from build123d import *

# Parameters (mm, degrees)
F1_DEPTH = 27.7749
F2_R     = 6.604
F4_D     = 6.604


with BuildPart() as f1:
    # F0 (on Right) → F1 (new body, symmetric)
    with BuildSketch(Plane.YZ):
        Polygon((77.47, 13.716), (0, 8.001), (0, 0), (77.47, 0), align=None)
    extrude(amount=F1_DEPTH, both=True)

    # F2
    f2_edges = [f1.edges().sort_by_distance(p)[0] for p in [
        (27.7749, 0, 4.0005),
        (27.7749, 77.47, 6.858),
        (-27.7749, 77.47, 6.858),
        (-27.7749, 0, 4.0005),
    ]]
    fillet(f2_edges, radius=F2_R)

    # F4 (through all)
    with Locations(Plane(origin=(0, 0, 0), x_dir=(1, 0, 0), z_dir=(0, 0, -1))):
        with Locations((22.0599, -5.715), (-22.0599, -5.715), (22.0599, -71.755), (-22.0599, -70.866)):
            Hole(F4_D / 2)


solid = f1.part
Geometry check sheet. Reference: the model listing, model coordinates, mm. Give positions to 0.01 mm unless a question says otherwise; leave off trailing zeros. Order: outer loops, then holes, each group sorted by start corner. A loop starts at its lowest first (then second) coordinate and runs counter-clockwise, first axis right, second up.
1. Sectioned sample at A-A (x = 23.5). Record the boundary of the cut face in (y, z).
Completed:
outline: (0.42, 0) - (2.74, 0) - (2.74, 8.2) - (0.42, 8.03) - close; (8.69, 0) - (68.78, 0) - (68.78, 13.08) - (8.69, 8.64) - close; (74.73, 0) - (77.05, 0) - (77.05, 13.68) - (74.73, 13.51) - close
2. Scan lines: line 1 (Y direction, x = 24, z = 2.75); line 2 (Y direction, x = -20, z = 3.75); line 3 (X direction, y = 73, z = 10.75). Record each from-to range of solid material in increasing order.
Completed:
line 1: y = 0.64 to 3.04, 8.39 to 69.08, 74.43 to 76.83
line 2: y = 0 to 3.13, 8.3 to 68.29, 73.45 to 77.47
line 3: x = -27.42 to -24.58, -19.54 to 19, 25.12 to 27.42
3. Sectioned sample at B-B (y = 7.5). Record the boundary of the cut face in (x, z).
Completed:
outline: (-27.77, 0) - (-24.84, 0) - (-24.84, 8.55) - (-27.77, 8.55) - close; (-19.28, 0) - (19.28, 0) - (19.28, 8.55) - (-19.28, 8.55) - close; (24.84, 0) - (27.77, 0) - (27.77, 8.55) - (24.84, 8.55) - close
4. Depth check by flat-ended pin: pin 1 (10.5 mm diameter, centred on x = -22.06, y = 5.72, fed in from +Z); pin 2 (5 mm diameter, centred on x = 12.5, y = 18.5, fed in from -Z); pin 3 (5.5 mm diameter, centred on x = -22.06, y = 70.87, fed in from +Z); pin 4 (1.5 mm diameter, centred on x = -1, y = 58, fed in from +Z) (3 decimals). Enter the tip coordinate at first touch or a pass-through.
Completed:
pin 1: stops at z = 8.81
pin 2: stops at z = 0
pin 3: passes through
pin 4: stops at z = 12.335
5. Draft check along X on faces 1 (the face through (0, 0, 4)), 2 (the face through (-25.11, 72.13, 6.86)), 3 (the face through (22.776, 74.978, 6.889)), 4 (the face through (25.789, 75.587, 6.954)). Enter one of: pulls with the +X half, pulls with the -X half, needs draft (parallel to the pull), parting line crosses it, or undercut.
Completed:
face 1: needs draft
face 2: undercut
face 3: undercut
face 4: pulls with the +X half
6. Sectioned sample at C-C (z = 11.5). Record the boundary of the cut face in (x, y) (3 decimals).
Completed:
outline: (-27.775, 47.431) - (27.775, 47.431) - (27.775, 70.866) arc R6.604 ccw to (21.171, 77.47) - (-21.171, 77.47) arc R6.604 ccw to (-27.775, 70.866) - close; hole circle Ø6.604 at (-22.06, 70.866); hole circle Ø6.604 at (22.06, 71.755)
7. Sectioned sample at D-D (z = 5.5). Record the boundary of the cut face in (x, y) (3 decimals), then the cut area to 3 significant figures.
Completed:
outline: (-27.775, 6.604) arc R6.604 ccw to (-21.171, 0) - (21.171, 0) arc R6.604 ccw to (27.775, 6.604) - (27.775, 70.866) arc R6.604 ccw to (21.171, 77.47) - (-21.171, 77.47) arc R6.604 ccw to (-27.775, 70.866) - close; hole circle Ø6.604 at (-22.06, 5.715); hole circle Ø6.604 at (-22.06, 70.866); hole circle Ø6.604 at (22.06, 5.715); hole circle Ø6.604 at (22.06, 71.755)
area: 4,130 mm2
